from build123d import *

# Parameters (mm, degrees)
LM8UU_CEN_X_Y_INT_R           = 4
LM8UU_CEN_X_Y_INT_DEPTH       = 27
LM8UU_CEN_X_Y_INT_PITCH_ANGLE = 90
LM8UU_CEN_X_Y_EXT_R           = 8
LM8UU_CEN_X_Y_EXT_DEPTH       = 25
LM8UU_CEN_X_Y_EXT_PITCH_ANGLE = 90


with BuildPart() as lm8uu_cen_x_y_int:
    # lm8uu_cen_x_y_int → lm8uu_cen_x_y_int (new body)
    with BuildSketch(Plane.XY):
        Circle(LM8UU_CEN_X_Y_INT_R)
    extrude(amount=LM8UU_CEN_X_Y_INT_DEPTH)


with BuildPart() as lm8uu_cen_x_y_int_1:
    # lm8uu_cen_x_y_int pitch: moved
    add(lm8uu_cen_x_y_int.part.rotate(Axis((0, 0, 0), (0, 1, 0)), LM8UU_CEN_X_Y_INT_PITCH_ANGLE))


with BuildPart() as lm8uu_cen_x_y_int_2:
    # lm8uu_cen_x_y_int placement: moved
    add(lm8uu_cen_x_y_int_1.part.moved(Location((-13.5, 0, 0))))


with BuildPart() as obj1:
    # lm8uu_cen_x_y_ext → lm8uu_cen_x_y_ext (new body)
    with BuildSketch(Plane.XY):
        Circle(LM8UU_CEN_X_Y_EXT_R)
    extrude(amount=LM8UU_CEN_X_Y_EXT_DEPTH)


with BuildPart() as obj1_1:
    # lm8uu_cen_x_y_ext pitch: moved
    add(obj1.part.rotate(Axis((0, 0, 0), (0, 1, 0)), LM8UU_CEN_X_Y_EXT_PITCH_ANGLE))


with BuildPart() as obj1_2:
    # lm8uu_cen_x_y_ext placement: moved
    add(obj1_1.part.moved(Location((-12.5, 0, 0))))

    # lm8uu_cen_x_y: cut lm8uu_cen_x_y_int
    add(lm8uu_cen_x_y_int_2.part, mode=Mode.SUBTRACT)


with BuildPart() as obj1_3:
    # lm8uu_cen_x_y placement: moved
    add(obj1_2.part.moved(Location((17.25, 32.5, 0))))


with BuildPart() as obj1_4:
    # Clone029 placement: moved
    add(obj1_3.part.moved(Location((0, -65, 0))))


solid = obj1_4.part
Geometry: final body of the model. Coordinates: model frame, mm. Coordinates: 2 decimals unless noted, no trailing zeros. Order: outer loops, then holes, each group sorted by start corner. A loop starts at its lowest first (then second) coordinate and runs counter-clockwise, first axis right, second up.
1) Section A-A (z = 0). Return loops of the section in (x, y), then the cut area to 3 significant figures.
Result sheet:
outline: (4.75, -40.5) - (29.75, -40.5) - (29.75, -36.5) - (4.75, -36.5) - close; (4.75, -28.5) - (29.75, -28.5) - (29.75, -24.5) - (4.75, -24.5) - close
area: 200 mm2
2) Draft query along X for faces 1 (the flat face through (4.75, -34, 4)), 2 (the flat face through (29.75, -34, 4)), 3 (the cylindrical face through (17.075, -24.568, 1.041)). Return one class per face: released by +X, released by -X, zero draft, split by the parting line, or undercut.
Result sheet:
face 1: released by -X
face 2: released by +X
face 3: zero draft
3) Ray query, probe 1 along Y at (x, z) = (12, 0); probe 2 along Y at (x, z) = (6, 1.75); probe 3 along Z at (x, y) = (15, -35.75). Return the intervals inside material, ascending.
Result sheet:
probe 1: y = -40.5 to -36.5, -28.5 to -24.5
probe 2: y = -40.31 to -36.1, -28.9 to -24.69
probe 3: z = -7.31 to -2.33, 2.33 to 7.31
4) First-contact query: P1, Ø2, axis at x = 10, z = 2, coming from the +Y side; P2, Ø5, axis at x = 15.5, y = -28, coming from the +Z side; P3, Ø1, axis at x = 10.5, z = 3, coming from the +Y side; P4, Ø6.5, axis at y = -32.5, z = 0, coming from the -X side. Flat tips, straight axial feed; report the tip coordinate or a pass-through.
Result sheet:
P1: stops at y = -24.56
P2: stops at z = 7.75
P3: stops at y = -24.9
P4: passes through
5) Section B-B (y = -32.5). Return loops of the section in (x, z).
Result sheet:
outline: (4.75, -8) - (29.75, -8) - (29.75, -4) - (4.75, -4) - close; (4.75, 4) - (29.75, 4) - (29.75, 8) - (4.75, 8) - close
6) Section C-C (x = 7). Return loops of the section in (y, z).
Result sheet:
outline: circle Ø16 at (-32.5, 0); hole circle Ø8 at (-32.5, 0)
7) Section D-D (z = -4.75). Return loops of the section in (x, y).
Result sheet:
outline: (4.75, -38.94) - (29.75, -38.94) - (29.75, -26.06) - (4.75, -26.06) - close
